Autodesk Inventor part; units mm, degrees
ref_plane "YZ Plane" through (0, 0, 0) normal (1, 0, 0) x (0, 1, 0)
ref_plane "XZ Plane" through (0, 0, 0) normal (0, 1, 0) x (-1, 0, 0)
ref_plane "XY Plane" through (0, 0, 0) normal (0, 0, 1) x (1, 0, 0)
sketch "Sketch1" plane through (0, 0, 0) normal (0, 0, 1) x (1, 0, 0)
  line L0 (0, 0) -> (90, 0)
  line L1 (90, 0) -> (90, 68)
  line L2 (90, 68) -> (0, 68)
  line L3 (0, 68) -> (0, 0)
  dimension "d0" = 90
  dimension "d1" = 68
extrude "Extrusion1" add sketch "Sketch1" along normal blind 2
sketch "Sketch2" plane through (0, 0, 2) normal (0, 0, 1) x (1, 0, 0)
  line L0 (90, 68) -> (0, 68)
  line L1 (0, 68) -> (90, 68)
  line L2 (90, 68) -> (90, 0)
  line L3 (90, 0) -> (0, 0)
  line L4 (0, 0) -> (0, 68)
  line L5 (2, 66) -> (88, 66)
  line L6 (88, 66) -> (88, 2)
  line L7 (88, 2) -> (2, 2)
  line L8 (2, 2) -> (2, 66)
  dimension "d4" = 2
  dimension "d5" = 2
  dimension "d6" = 2
  dimension "d7" = 2
extrude "Extrusion2" add sketch "Sketch2" along normal blind 10
sketch "Sketch3" plane through (0, 0, 2) normal (0, 0, 1) x (1, 0, 0)
  line L0 (6, 63.2) -> (86, 63.2)
  line L1 (86, 63.2) -> (86, 4.8)
  line L2 (86, 4.8) -> (6, 4.8)
  line L3 (4, 21.3) -> (4, 57.2)
  line L4 (2, 66) -> (88, 66)
  line L5 (0, 0) -> (90, 0)
  line L6 (90, 68) -> (0, 68)
  line L7 (88, 2) -> (2, 2)
  line L8 (2, 2) -> (2, 66)
  line L9 (88, 66) -> (88, 2)
  line L10 (47.8, 63.2) -> (50.703, 63.2)
  line L11 (50.703, 63.2) -> (50.703, 64.6)
  line L12 (50.703, 64.6) -> (47.8, 64.6)
  line L13 (47.8, 64.6) -> (47.8, 63.2)
  circle A0 centre (82, 59.7) radius 1.5
  line L14 (4, 57.2) -> (6, 59.2)
  line L15 (4, 57.2) -> (6.8284, 57.2) construction
  line L16 (6, 59.2) -> (6, 63.2)
  line L17 (4, 21.3) -> (6, 19.3)
  line L18 (4, 21.3) -> (6.8284, 21.3) construction
  line L19 (6, 19.3) -> (6, 4.8)
  circle A1 centre (8.75, 53.95) radius 1.25
  circle A2 centre (8.75, 25.95) radius 1.25
  line L20 (86.5, 63.7) -> (5.5, 63.7)
  line L21 (5.5, 63.7) -> (5.5, 59.4071)
  line L22 (5.5, 59.4071) -> (3.5, 57.4071)
  line L23 (3.5, 57.4071) -> (3.5, 21.0929)
  line L24 (3.5, 21.0929) -> (5.5, 19.0929)
  line L25 (5.5, 19.0929) -> (5.5, 4.3)
  line L26 (5.5, 4.3) -> (86.5, 4.3)
  line L27 (86.5, 4.3) -> (86.5, 63.7)
  circle A3 centre (82, 8.8) radius 1.5
  dimension "d11" = 58.4
  dimension "d12" = 2.8
  dimension "d14" = 64
  dimension "d18" = 2
  dimension "d19" = 86
  dimension "d20" = 38.2
  dimension "d21" = 1.4
  dimension "d22" = 3
  dimension "d23" = 3.5
  dimension "d24" = 4
  dimension "d25" = 45
  dimension "d26" = 4
  dimension "d28" = 45
  dimension "d30" = 2
  dimension "d31" = 2
  dimension "d32" = 82
  dimension "d33" = 2.5
  dimension "d34" = 4.75
  dimension "d36" = 2.5
  dimension "d38" = 25.5
  dimension "d39" = 8
  dimension "d40" = 14.5
  dimension "d41" = 39.9
  dimension "d42" = 0.5
  dimension "d45" = 3
  dimension "d47" = 2.5
extrude "Extrusion3" add sketch "Sketch3" along normal blind 5
fillet "Fillet1" radius 1 4 edges at (7.5, 53.95, 7) (7.5, 25.95, 7) (80.5, 59.7, 7) (80.5, 8.8, 7)
fillet "Fillet2" radius 0.5 12 edges at (26.65, 63.7, 7) (5.5, 61.5536, 7) (4.5, 58.4071, 7) (3.5, 39.25, 7) (4.5, 20.0929, 7) (5.5, 11.6964, 7) (46, 4.3, 7) (86.5, 34, 7) (68.6015, 63.7, 7) (49.2515, 64.6, 7) (50.703, 64.15, 7) (47.8, 64.15, 7)
equation "\"d12\" = -0.5 * d11 + 0.5 * d14"
equation "\"d18\" = -0.5 * d10 + 0.5 * d19"
properties part number "Lådaprototyp"
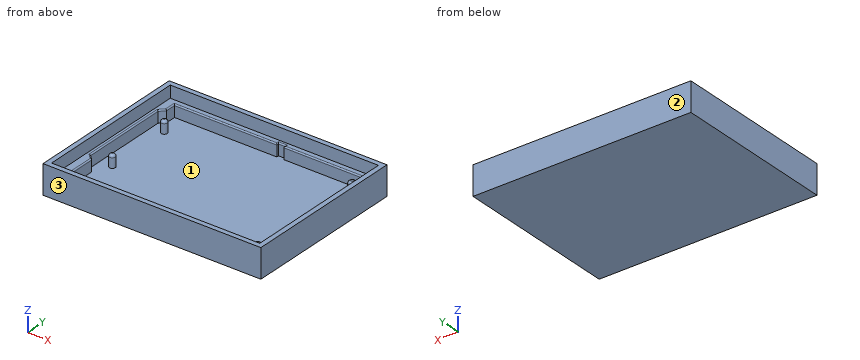
Design review of the part built by this model. Coordinates are the model's own, in mm. Face numbers are marked on the shaded views. Coordinates: 2 decimals unless noted, no trailing zeros. Write each loop counter-clockwise with the first axis right and the second up, starting at its lowest first coordinate (ties: lowest second). Pieces come first, ordered by that corner, then holes. Notation, with made-up numbers: M 88.5,89 L 129.5,89 A25 cw 129.5,101 Z; hole C -23.5,-6.5 d4. An arc over 180 degrees is marked long. Answer as a JSON object with one key per item and string values.
Item 1: Wall thickness on probe 1 along X at (y, z) = (59.5, 5); probe 2 along X at (y, z) = (35.5, 7.5); probe 3 along X at (y, z) = (49, 3.5): over which ranges is each line inside the solid? List them lowest first.
Outcome:
{"probe 1": "0 to 5.5, 80.51 to 83.49, 86.5 to 90", "probe 2": "0 to 2, 88 to 90", "probe 3": "0 to 3.5, 86.5 to 90"}
Item 2: Draft analysis for pull direction Y (two halves, no side actions). For the marked faces 1, 2 and 3, state which applies: pulls with the +Y half, pulls with the -Y half, needs draft (parallel to the pull), parting line crosses it, or undercut.
Outcome:
{"face 1": "undercut", "face 2": "pulls with the +Y half", "face 3": "pulls with the -Y half"}
Item 3: Add section A-A, the plane z = 5. Give the boundary of the cut face in (x, y), and give its area (3 significant figures).
Outcome:
{"outline": "M 0,0 L 90,0 L 90,68 L 0,68 Z; C 8.75,25.95 d2.5; C 8.75,53.95 d2.5; C 82,8.8 d3; C 82,59.7 d3; hole M 3.5,21.09 L 5.5,19.09 L 5.5,4.3 L 86.5,4.3 L 86.5,63.7 L 50.7,63.7 L 50.7,64.6 L 47.8,64.6 L 47.8,63.7 L 5.5,63.7 L 5.5,59.41 L 3.5,57.41 Z", "area": "1,250 mm²"}
Item 4: Add section B-B, the plane y = 34. Give the boundary of the cut face in (x, z), and give its area (3 significant figures).
Outcome:
{"outline": "M 0,0 L 90,0 L 90,12 L 88,12 L 88,7 L 87,7 A0.5 ccw 86.5,6.5 L 86.5,2 L 3.5,2 L 3.5,6.5 A0.5 ccw 3,7 L 2,7 L 2,12 L 0,12 Z", "area": "235 mm²"}
Item 5: Insertion check: pin 1 Ø0.6 at (x, y) = (8.5, 54) entering from +Z; pin 2 Ø1.5 at (x, z) = (26, 8.5) entering from -Y; pin 3 Ø1.5 at (x, y) = (30.5, 59) entering from +Z. Each pin has a flat end and moves straight along its axis. Give the tip position at first contact, or say it passes through.
Outcome:
{"pin 1": "z = 7", "pin 2": "y = 0", "pin 3": "z = 2"}
Item 6: Add section C-C, the plane x = 26.5. Give the boundary of the cut face in (y, z).
Outcome:
{"outline": "M 0,0 L 68,0 L 68,12 L 66,12 L 66,7 L 64.2,7 A0.5 ccw 63.7,6.5 L 63.7,2 L 4.3,2 L 4.3,6.5 A0.5 ccw 3.8,7 L 2,7 L 2,12 L 0,12 Z"}
